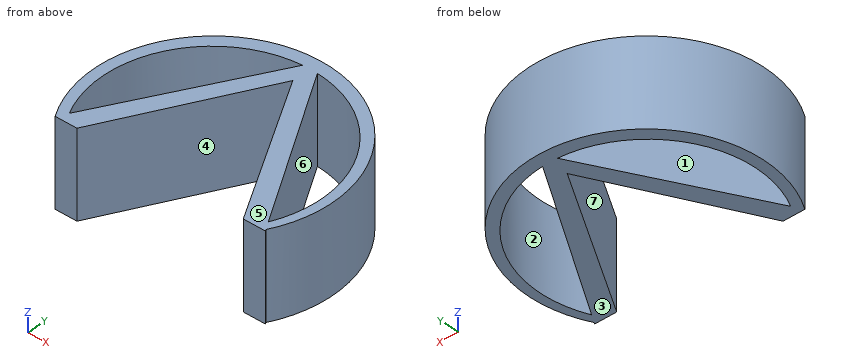
from build123d import *

# Parameters (mm, degrees)
EXTRUDE_1_DEPTH = 50


with BuildPart() as part:
    # 草图3 → 凸台-拉伸1 (new body)
    with BuildSketch(Plane.XY):
        with BuildLine():
            ThreePointArc((-58.793503257, -35.392156003), (-2.246555748, 68.568474272), (59.534802182, -32.36929731))
            Line((59.534802182, -32.36929731), (60.047257822, -33.220589397))
            Line((60.047257822, -33.220589397), (47.551744298, -33.448918799))
            Line((47.551744298, -33.448918799), (-1.253754565, 50.734372928))
            Line((-1.253754565, 50.734372928), (-46.430511789, -35.166248165))
            Line((-46.430511789, -35.166248165), (-58.793503257, -35.392156003))
        make_face()
        with BuildLine():
            Line((-5.324718346, 61.254350615), (-55.742028798, -29.87652016))
            ThreePointArc((-55.742028798, -29.87652016), (-54.854751969, 29.144492628), (-5.324718346, 61.254350615))
        make_face(mode=Mode.SUBTRACT)
        with BuildLine():
            Line((56.759373511, -27.75875099), (3.086082061, 61.403402212))
            ThreePointArc((3.086082061, 61.403402212), (53.687117349, 31.127868506), (56.759373511, -27.75875099))
        make_face(mode=Mode.SUBTRACT)
    extrude(amount=EXTRUDE_1_DEPTH)


solid = part.part
For this review, take the finished solid that the model builds, in its own axes (mm). Face numbers are marked on the shaded views. A direction names the side the tool comes from. Coordinates: 2 decimals unless noted, no trailing zeros. Loops run counter-clockwise (first coordinate to the right, second up) from the corner with the lowest first, then second, coordinate; pieces in that order, holes last. Notation, with made-up numbers: (-12.5, -15) - (34.5, -15) arc R25 cw to (34.5, -2) - close; hole circle Ø11 at (13, 43). An arc over 180 degrees is marked (long way). Use a Markdown table: item, result. Add a question column.
Item 1: We need section C-C (z = 27). Give the boundary of the cut face in (x, y), and give its area (3 significant figures).
Item 2: We need section D-D (y = 9.5). Give the boundary of the cut face in (x, z), and give its area (3 significant figures).
Item 3: Tool access review of the marked faces 5, 6 and 7: name each direction out of +Z, -Z, +X, -X, +Y, -Y from which nothing blocks a thin tool from reaching the whole face with its end or side.
Item 4: Mouldability with a two-part tool opening along Y and no side actions: class the marked faces 1, 2, 3 and 4 as pulls with the +Y half, pulls with the -Y half, needs draft (parallel to the pull), parting line crosses it, or undercut.
Item 5: For line 1 (X direction, y = 39, z = 18.5); line 2 (X direction, y = 48.5, z = 10); line 3 (X direction, y = 56.5, z = 3.5), list the stretches that pass through material, from the lowest coordinate up.
Item 6: We need section A-A (y = 56.5). Give the boundary of the cut face in (x, z), and give its area (3 significant figures).
Item 7: Insertion check: pin 1 Ø3 at (x, z) = (19, 17.5) entering from +Y; pin 2 Ø4 at (x, z) = (44.5, 23) entering from -Y; pin 3 Ø5 at (y, z) = (21.5, 36) entering from -X; pin 4 Ø12 at (x, y) = (-39.5, 17.5) entering from +Z. Each pin has a flat end and moves straight along its axis. Give the tip position at first contact, or say it passes through.
Item 8: We need section B-B (x = -48.5). Give the boundary of the cut face in (y, z).
Results list:
| question | item | result |
|---|---|---|
| 1 | outline | (-58.79, -35.39) - (-46.43, -35.17) - (-1.25, 50.73) - (47.55, -33.45) - (60.05, -33.22) - (59.53, -32.37) arc R68.33 ccw (long way) to start; hole (-55.74, -29.88) - (-5.32, 61.25) arc R62.68 ccw to start; hole (3.09, 61.4) - (56.76, -27.76) arc R62.68 ccw to start |
| 1 | area | 3,790 mm^2 |
| 2 | outline | (-68.2, 0) - (-61.77, 0) - (-61.77, 50) - (-68.2, 50) - close; (-33.96, 0) - (-22.94, 0) - (-22.94, 50) - (-33.96, 50) - close; (22.65, 0) - (34.33, 0) - (34.33, 50) - (22.65, 50) - close; (61.75, 0) - (67.2, 0) - (67.2, 50) - (61.75, 50) - close |
| 2 | area | 1,730 mm^2 |
| 3 | face 5 | +Z, +X, -X, +Y, -Y |
| 3 | face 6 | +Z, -Z |
| 3 | face 7 | +Z, -Z, -Y |
| 4 | face 1 | undercut |
| 4 | face 2 | undercut |
| 4 | face 3 | needs draft |
| 4 | face 4 | pulls with the -Y half |
| 5 | line 1 | x = -56.79 to -48.1, -17.64 to -7.43, 5.55 to 16.57, 48.08 to 55.79 |
| 5 | line 2 | x = -48.9 to -38.2, -12.38 to -2.43, 0.04 to 10.85, 38.18 to 47.89 |
| 5 | line 3 | x = -39.31 to -24.5, -7.96 to 6.04, 24.47 to 38.31 |
| 6 | outline | (-39.31, 0) - (-24.5, 0) - (-24.5, 50) - (-39.31, 50) - close; (-7.96, 0) - (6.04, 0) - (6.04, 50) - (-7.96, 50) - close; (24.47, 0) - (38.31, 0) - (38.31, 50) - (24.47, 50) - close |
| 6 | area | 2,130 mm^2 |
| 7 | pin 1 | stops at y = 66.18 |
| 7 | pin 2 | stops at y = -31.63 |
| 7 | pin 3 | stops at x = -66.21 |
| 7 | pin 4 | passes through |
| 8 | outline | (-35.2, 0) - (-16.79, 0) - (-16.79, 50) - (-35.2, 50) - close; (38.52, 0) - (48.89, 0) - (48.89, 50) - (38.52, 50) - close |
